```python
from build123d import *

# Parameters (mm, degrees)
SKETCH1_W           = 67
SKETCH1_H           = 130
SKETCH1_W_2         = 61
SKETCH1_H_2         = 124
BOSS_EXTRUDE1_DEPTH = 10
SKETCH2_W           = 67
SKETCH2_H           = 130
SKETCH2_W_2         = 26.1
SKETCH2_H_2         = 72.5
SKETCH2_W_3         = 7
SKETCH2_H_3         = 11.999999998
BOSS_EXTRUDE2_DEPTH = 2
SKETCH3_R           = 2
CUT_EXTRUDE1_DEPTH  = 78.042717027
SKETCH4_R           = 2.2
CUT_EXTRUDE2_DEPTH  = 78.042717027


with BuildPart() as part:
    # Sketch1 → Boss-Extrude1 (new body)
    with BuildSketch(Plane.XY):
        with Locations((0, -3.332497736)):
            Rectangle(SKETCH1_W, SKETCH1_H)
        with Locations((0, -3.332497736)):
            Rectangle(SKETCH1_W_2, SKETCH1_H_2, mode=Mode.SUBTRACT)
    extrude(amount=BOSS_EXTRUDE1_DEPTH)

    # Sketch2 → Boss-Extrude2 (add)
    with BuildSketch(Plane.XY.offset(10)):
        with Locations((0, -3.332497736)):
            Rectangle(SKETCH2_W, SKETCH2_H)
        with Locations((-2.35, -17.717502264)):
            Rectangle(SKETCH2_W_2, SKETCH2_H_2, mode=Mode.SUBTRACT)
        with Locations((-26, -49.667502265)):
            Rectangle(SKETCH2_W_3, SKETCH2_H_3, mode=Mode.SUBTRACT)
    extrude(amount=BOSS_EXTRUDE2_DEPTH)

    # Sketch3 → Cut-Extrude1 (cut, through all)
    with BuildSketch(Plane.XY.offset(12)):
        with Locations((23.09645, -52.119552264)):
            Circle(SKETCH3_R)
        with Locations((23.09645, -44.115452264)):
            Circle(SKETCH3_R)
        with Locations((18.715647246, -35.063805606)):
            Circle(SKETCH3_R)
        with Locations((23.09645, -26.115452264)):
            Circle(SKETCH3_R)
        with Locations((23.09645, -18.115452264)):
            Circle(SKETCH3_R)
        with Locations((25.496463554, -35.066106361)):
            Circle(SKETCH3_R)
    extrude(amount=-CUT_EXTRUDE1_DEPTH, mode=Mode.SUBTRACT)

    # Sketch4 → Cut-Extrude2 (cut, through all)
    with BuildSketch(Plane.XY.offset(12)):
        with Locations((-29, 57.167502264)):
            Circle(SKETCH4_R)
        with Locations((29, 57.167502264)):
            Circle(SKETCH4_R)
        with Locations((-29, -63.832497736)):
            Circle(SKETCH4_R)
        with Locations((29, -63.832497736)):
            Circle(SKETCH4_R)
    extrude(amount=-CUT_EXTRUDE2_DEPTH, mode=Mode.SUBTRACT)


solid = part.part
```
Work out the finished part from the listing and answer in its coordinate system (mm). A direction names the side the tool comes from. Round coordinates to 2 decimals unless told otherwise and drop trailing zeros. Loops run counter-clockwise (first coordinate to the right, second up) from the corner with the lowest first, then second, coordinate; pieces in that order, holes last.
(1) The part is cut by section A-A, the plane y = 12. Give the vertices of the cut face in (x, z).
Computed values:
outline: (-33.5, 0) - (-30.5, 0) - (-30.5, 10) - (-15.4, 10) - (-15.4, 12) - (-33.5, 12) - close; (10.7, 10) - (30.5, 10) - (30.5, 0) - (33.5, 0) - (33.5, 12) - (10.7, 12) - close
(2) Each of these flat-tipped pins is pushed along its axis until it touches: P1, Ø2.5, axis at x = 25.5, y = -35.07, coming from the -Z side; P2, Ø1, axis at x = 1.5, y = 45.5, coming from the -Z side. Where does it stop, or does it pass through?
Computed values:
P1: passes through
P2: stops at z = 10
(3) The mould has two halves that part along Y. Classify faces 1 (the flat face through (14, -2, 12)), 2 (the flat face through (0, 61.668, 6)), 3 (the cylindrical face through (22.663, -46.068, 11.014)): pulls with the +Y half, pulls with the -Y half, needs draft (parallel to the pull), parting line crosses it, or undercut.
Computed values:
face 1: needs draft
face 2: pulls with the +Y half
face 3: undercut
(4) For faces 4 (the cylindrical face through (30.02, -65.78, 7.42)), 5 (the flat face through (0, 58.668, 5)), determine the directions among +Z, -Z, +X, -X, +Y, -Y from which every point of the face is accessible in a straight line to the end or side of a thin tool.
Computed values:
face 4: +Z, -Z
face 5: -Z
(5) The part is cut by section D-D, the plane x = 1. Give the vertices of the cut face in (y, z), and give its area (3 significant figures).
Computed values:
outline: (-68.33, 0) - (-65.33, 0) - (-65.33, 10) - (-53.97, 10) - (-53.97, 12) - (-68.33, 12) - close; (18.53, 10) - (58.67, 10) - (58.67, 0) - (61.67, 0) - (61.67, 12) - (18.53, 12) - close
area: 175 mm2
(6) The part is cut by section C-C, the plane z = 6.5. Give the vertices of the cut face in (x, y), and give its area (3 significant figures).
Computed values:
outline: (-33.5, -68.33) - (33.5, -68.33) - (33.5, 61.67) - (-33.5, 61.67) - close; hole (-30.5, -62.22) arc R2.2 ccw (long way) to (-27.39, -65.33) - (27.39, -65.33) arc R2.2 ccw (long way) to (30.5, -62.22) - (30.5, 55.56) arc R2.2 ccw (long way) to (27.39, 58.67) - (-27.39, 58.67) arc R2.2 ccw (long way) to (-30.5, 55.56) - close
area: 1,130 mm2
(7) The part is cut by section B-B, the plane x = 29. Give the vertices of the cut face in (y, z).
Computed values:
outline: (-68.33, 0) - (-66.03, 0) - (-66.03, 12) - (-68.33, 12) - close; (-61.63, 10) - (54.97, 10) - (54.97, 12) - (-61.63, 12) - close; (59.37, 0) - (61.67, 0) - (61.67, 12) - (59.37, 12) - close
(8) Find the intervals of material crossed by L1, parallel to Y at x = 9, z = 6.75; L2, parallel to X at y = -9.5, z = 5.5; L3, parallel to X at y = 9, z = 10.25, in increasing order.
Computed values:
L1: y = -68.33 to -65.33, 58.67 to 61.67
L2: x = -33.5 to -30.5, 30.5 to 33.5
L3: x = -33.5 to -15.4, 10.7 to 33.5
